Input: dimensioned drawing with shaded views. Units: mm. Origin: part minimum x, y, z. A direction names the side the tool comes from. Round coordinates to 2 decimals unless told otherwise and drop trailing zeros. Order: outer loops, then holes, each group sorted by start corner. A loop starts at its lowest first (then second) coordinate and runs counter-clockwise, first axis right, second up. Notation, with made-up numbers: (-39.5, -39) - (-18.5, -39) arc R34 ccw to (-18.5, -5) - close; hole circle Ø2 at (71.25, 87). An arc over 180 degrees is marked (long way). Return JSON: item names as keys, results as strings. Group by question number.
1) Section A-A, the plane y = 62.5. Return loops of the section in (x, z), plus the area to 3 significant figures.
2) Mould query, pull axis X, two halves, no side actions, for the marked faces 3, 4, 5 and 6. Classes: pulls with the +X half, pulls with the -X half, needs draft (parallel to the pull), parting line crosses it, or undercut.
3) Ray query, line 1 (X direction, y = 10.5, z = 173.5); line 2 (Y direction, x = 41, z = 84.5). Return the intervals inside material, ascending. Write a range as from..to.
4) Access query for the marked faces 1 and 2. Directions: +Z, -Z, +X, -X, +Y, -Y. A direction counts if a zero-diameter tool reaches every point of the face in a straight line with its end or side. Return the directions, or none.
5) Contact query for a flat-ended pin moving along its axis: P1, Ø12, axis at y = 23, z = 134, coming from the -X side. Output: stop coordinate, or through.
6) Section C-C, the plane x = 45. Return loops of the section in (y, z).
7) Section B-B, the plane z = 113.5. Return loops of the section in (x, y), plus the area to 3 significant figures.
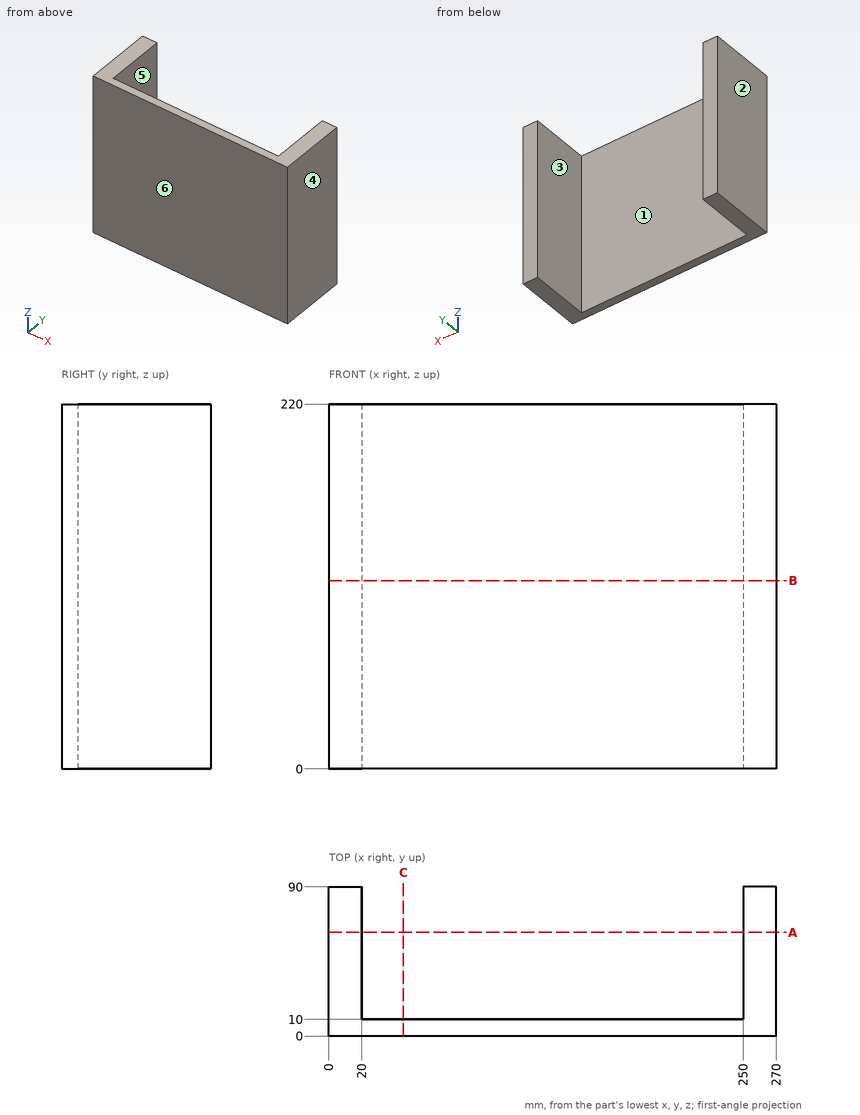
Geometry check:
{
 "1": {"outline": "(0, 0) - (20, 0) - (20, 220) - (0, 220) - close; (250, 0) - (270, 0) - (270, 220) - (250, 220) - close", "area": "8,800 mm2"},
 "2": {"face 3": "undercut", "face 4": "pulls with the +X half", "face 5": "undercut", "face 6": "needs draft"},
 "3": {"line 1": "0..20, 250..270", "line 2": "0..10"},
 "4": {"face 1": "+Z, -Z, +Y", "face 2": "+Z, -Z, -X, +Y, -Y"},
 "5": {"P1": "x = 0"},
 "6": {"outline": "(0, 0) - (10, 0) - (10, 220) - (0, 220) - close"},
 "7": {"outline": "(0, 0) - (270, 0) - (270, 90) - (250, 90) - (250, 10) - (20, 10) - (20, 90) - (0, 90) - close", "area": "5,900 mm2"}
}
